from build123d import *

# Parameters (mm, degrees)
F0_W     = 1450
F0_H     = 650
F1_DEPTH = 30
F2_R     = 2
F3_W     = 1386
F3_H     = 586
F4_DEPTH = 25
F5_R     = 5


with BuildPart() as f1:
    # F0 (on Top) → F1 (new body)
    with BuildSketch(Plane.XY):
        with Locations((725, 325)):
            Rectangle(F0_W, F0_H)
    extrude(amount=-F1_DEPTH)

    # F2
    f2_edges = [f1.edges().sort_by_distance(p)[0] for p in [
        (0, 650, -15),
        (725, 650, -30),
        (0, 325, -30),
        (725, 0, -30),
        (1450, 325, -30),
        (0, 325, 0),
        (725, 0, 0),
        (1450, 325, 0),
        (725, 650, 0),
        (0, 0, -15),
        (1450, 0, -15),
        (1450, 650, -15),
    ]]
    fillet(f2_edges, radius=F2_R)

    # F3 (on face) → F4 (cut)
    with BuildSketch(Plane(origin=(0, 0, -30), x_dir=(1, 0, 0), z_dir=(0, 0, -1))):
        with Locations((725, -325)):
            Rectangle(F3_W, F3_H)
    extrude(amount=-F4_DEPTH, mode=Mode.SUBTRACT)

    # F5
    f5_edges = [f1.edges().sort_by_distance(p)[0] for p in [
        (1418, 618, -17.5),
        (1418, 32, -17.5),
        (32, 32, -17.5),
        (32, 325, -30),
        (1418, 325, -30),
        (32, 618, -17.5),
        (725, 618, -30),
        (725, 32, -30),
    ]]
    fillet(f5_edges, radius=F5_R)


solid = f1.part
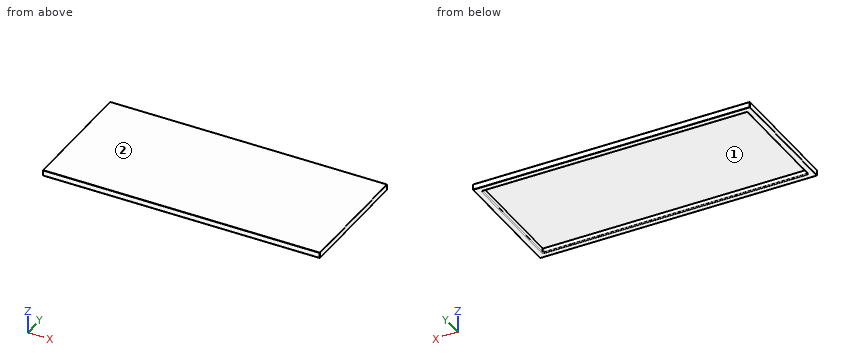
Could you check a few things on this model? Use its own coordinates, in mm. Face numbers are marked on the shaded views. Round coordinates to 2 decimals unless told otherwise and drop trailing zeros. Write each loop counter-clockwise with the first axis right and the second up, starting at its lowest first coordinate (ties: lowest second). Pieces come first, ordered by that corner, then holes. Notation, with made-up numbers: (77, -23) - (96, -23) arc R28 cw to (96, -1) - close; hole circle Ø11 at (44.25, -21). An arc over 180 degrees is marked (long way). Put each result on its own line as item: value. Start each with the question number.
(1) I want a section at B-B, the plane y = 347. Please give me the cut outline in (x, z), plus the area to 3 significant figures.
(2) I need wall thicknesses on probe 1 along Y at (x, z) = (728, -11.75); probe 2 along X at (y, z) = (250.5, -23); probe 3 along Y at (x, z) = (1269, -26.5). Which ranges of each line are inside material? Lowest first, please.
(3) Will this pin go through, and if not, where does the flat tip stop? pin 1 (2 mm diameter, centred on x = 578.5, y = 374.5, fed in from -Z).
(4) Thinking about a two-plate mould opening in Y: for the marked faces 1 and 2, which applies, released by +Y, released by -Y, zero draft, split by the parting line, or undercut?
(5) I want a section at A-A, the plane z = -9.75. Please give me the cut outline in (x, y), plus the area to 3 significant figures.
(6) I want a section at C-C, the plane x = 462. Please give me the cut outline in (y, z).
Here are the results:
1. outline: (0, -28) arc R2 ccw to (2, -30) - (27, -30) arc R5 ccw to (32, -25) - (32, -5) - (1418, -5) - (1418, -25) arc R5 ccw to (1423, -30) - (1448, -30) arc R2 ccw to (1450, -28) - (1450, -2) arc R2 ccw to (1448, 0) - (2, 0) arc R2 ccw to (0, -2) - close
1. area: 8,840 mm^2
2. probe 1: y = 0 to 32, 618 to 650
2. probe 2: x = 0 to 32, 1418 to 1450
2. probe 3: y = 0 to 31.77, 618.23 to 650
3. pin 1: stops at z = -5
4. face 1: undercut
4. face 2: zero draft
5. outline: (0, 2) arc R2 ccw to (2, 0) - (1448, 0) arc R2 ccw to (1450, 2) - (1450, 648) arc R2 ccw to (1448, 650) - (2, 650) arc R2 ccw to (0, 648) - close; hole (32, 37) arc R5 ccw to (37, 32) - (1413, 32) arc R5 ccw to (1418, 37) - (1418, 613) arc R5 ccw to (1413, 618) - (37, 618) arc R5 ccw to (32, 613) - close
5. area: 130,000 mm^2
6. outline: (0, -28) arc R2 ccw to (2, -30) - (27, -30) arc R5 ccw to (32, -25) - (32, -5) - (618, -5) - (618, -25) arc R5 ccw to (623, -30) - (648, -30) arc R2 ccw to (650, -28) - (650, -2) arc R2 ccw to (648, 0) - (2, 0) arc R2 ccw to (0, -2) - close
